from build123d import *

# Parameters (mm, degrees)
SALIENTE_EXTRUIR1_DEPTH = 20
CROQUIS2_R              = 1.75
SALIENTE_EXTRUIR2_DEPTH = 5
MATRIZL1_COUNT          = 2
MATRIZL1_PITCH          = 10
SALIENTE_EXTRUIR3_DEPTH = 3


with BuildPart() as part:
    # Croquis1 → Saliente-Extruir1 (new body)
    with BuildSketch(Plane(origin=(0, 0, 0), x_dir=(1, 0, 0), z_dir=(0, 1, 0))):
        with BuildLine():
            Line((-50.5, 0), (50.5, 0))
            Line((50.5, 0), (50.5, 7))
            Line((50.5, 7), (43.6, 7))
            ThreePointArc((43.6, 7), (31.822793565, 12.849892164), (29.368318159, 25.768846465))
            ThreePointArc((29.368318159, 25.768846465), (25.038732007, 51.41585196), (2.5, 64.397368307))
            Line((2.5, 64.397368307), (2.5, 60.381811917))
            ThreePointArc((2.5, 60.381811917), (0, 7.5), (-2.5, 60.381811917))
            Line((-2.5, 60.381811917), (-2.5, 64.397368307))
            ThreePointArc((-2.5, 64.397368307), (-25.038732007, 51.41585196), (-29.368318159, 25.768846465))
            ThreePointArc((-29.368318159, 25.768846465), (-31.822793565, 12.849892164), (-43.6, 7))
            Line((-43.6, 7), (-50.5, 7))
            Line((-50.5, 7), (-50.5, 0))
        make_face()
        with BuildLine():
            Line((14.186260959, 7), (32.013771293, 7))
            ThreePointArc((32.013771293, 7), (27.872929965, 11.516026639), (25.406103057, 17.124576229))
            ThreePointArc((25.406103057, 17.124576229), (20.433198062, 11.356360342), (14.186260959, 7))
        make_face(mode=Mode.SUBTRACT)
        with BuildLine():
            Line((-32.013771293, 7), (-14.186260959, 7))
            ThreePointArc((-14.186260959, 7), (-20.433198062, 11.356360342), (-25.406103057, 17.124576229))
            ThreePointArc((-25.406103057, 17.124576229), (-27.872929965, 11.516026639), (-32.013771293, 7))
        make_face(mode=Mode.SUBTRACT)
    extrude(amount=SALIENTE_EXTRUIR1_DEPTH)

    # Croquis2 → Saliente-Extruir2 (add)
    with BuildSketch(Plane.ZY.offset(-2.5)):
        with BuildLine():
            Line((-60.381811917, 20), (-60.381811917, 0))
            Line((-60.381811917, 0), (-71.739628608, 0))
            ThreePointArc((-71.739628608, 0), (-76.060720262, 15.678908346), (-60.381811917, 20))
        make_face()
        with Locations((-72.810720262, 10)):
            Circle(CROQUIS2_R, mode=Mode.SUBTRACT)
    saliente_extruir2 = extrude(amount=-SALIENTE_EXTRUIR2_DEPTH)

    # MatrizL1: Saliente-Extruir2 ×2
    with Locations(*[(-i * MATRIZL1_PITCH, 0, 0) for i in range(1, MATRIZL1_COUNT)]):
        add(saliente_extruir2)

    # Croquis3 → Saliente-Extruir3 (add)
    with BuildSketch(Plane(origin=(0, 0, 0), x_dir=(1, 0, 0), z_dir=(0, 1, 0))):
        with BuildLine():
            Line((-7.5, 70.792294373), (-7.5, 63.563490998))
            ThreePointArc((-7.5, 63.563490998), (-20.283716212, 56.7776394), (-28.5, 44.862780491))
            add(Edge.make_bspline(
                [(-7.5, 70.792294373), (-28.5, 65.390312314), (-28.5, 44.862780491)],
                knots=[4.978682998, 4.978682998, 4.978682998, 6.283185307, 6.283185307, 6.283185307], degree=2, weights=[1, 0.794719414, 1]))
        make_face()
        with BuildLine():
            Line((7.5, 70.792294373), (7.5, 63.563490998))
            ThreePointArc((7.5, 63.563490998), (20.283716212, 56.7776394), (28.5, 44.862780491))
            add(Edge.make_bspline(
                [(28.5, 44.862780491), (28.5, 65.390312314), (7.5, 70.792294373)],
                knots=[3.141592654, 3.141592654, 3.141592654, 4.446094963, 4.446094963, 4.446094963], degree=2, weights=[1, 0.794719414, 1]))
        make_face()
    extrude(amount=SALIENTE_EXTRUIR3_DEPTH)


solid = part.part
Work out the finished part from the listing and answer in its coordinate system (mm). A direction names the side the tool comes from. Round coordinates to 2 decimals unless told otherwise and drop trailing zeros. Write each loop counter-clockwise with the first axis right and the second up, starting at its lowest first coordinate (ties: lowest second). Pieces come first, ordered by that corner, then holes.
1) A cutting plane is placed at B-B (y = 10). Give the number of separate pieces and of enclosed holes in the cut face, plus the area to 3 significant figures.
2) The mould has two halves that part along X. Classify faces 6 (the cylindrical face through (-5.04, 10.08, -74.56)), 7 (the flat face through (50.5, 10, -3)), 8 (the cylindrical face through (20.512, 9.86, -11.428)): pulls with the +X half, pulls with the -X half, needs draft (parallel to the pull), parting line crosses it, or undercut.
3) A cutting plane is placed at D-D (y = 15.5). Give the vertices of the cut face in (x, z).
4) Given pin 1 Ø7.5 at (x, y) = (48.5, 11.5) entering from -Z; pin 2 Ø4 at (y, z) = (10, -72.81) entering from +X; pin 3 Ø10.5 at (x, z) = (20.5, -58.5) entering from +Y; pin 4 Ø2 at (y, z) = (10, -72.81) entering from +X, each flat-ended and moving along its own axis, determine where each tip first touches the part or whether it passes through.
5) A cutting plane is placed at A-A (z = -34). Give the vertices of the cut face in (x, y).
6) A tool of negligible diameter and unlimited length cuts with its end or side. For faces 1 (the flat face through (47, 10, -7)), 2 (the flat face through (-2.5, 11, -69)), 3 (the flat face through (7.5, 11, -71)), 4 (the cylindrical face through (1.13, 9.86, -7.524)), 5 (the flat face through (-7.5, 11, -71)), from which of +Z, -Z, +X, -X, +Y, -Y can it reach the whole face along a straight path? Write none if from no direction.
7) A cutting plane is placed at C-C (z = -14.5). Give the vertices of the cut face in (x, y), plus the area to 3 significant figures.
8) Straight lines are drawn through the part: line 1 (X direction, y = 12, z = -34); line 2 (X direction, y = 13.25, z = -9.5); line 3 (Y direction, x = 18.5, z = -6). For each, find the intervals that lie inside material, in ascending order.
Completed:
1. separate pieces: 3
1. enclosed holes: 2
1. area: 1,570 mm2
2. face 6: needs draft
2. face 7: pulls with the +X half
2. face 8: undercut
3. outline: (-50.5, -7) - (-43.6, -7) arc R14.78 cw to (-29.37, -25.77) arc R30.5 ccw to (-7.5, -63.56) - (-7.5, -76.16) - (-2.5, -76.16) - (-2.5, -60.38) arc R26.5 cw (long way) to (2.5, -60.38) - (2.5, -76.16) - (7.5, -76.16) - (7.5, -63.56) arc R30.5 ccw to (29.37, -25.77) arc R14.78 cw to (43.6, -7) - (50.5, -7) - (50.5, 0) - (-50.5, 0) - close; hole (-32.01, -7) arc R18.78 cw to (-25.41, -17.12) arc R30.5 cw to (-14.19, -7) - close; hole (14.19, -7) arc R30.5 cw to (25.41, -17.12) arc R18.78 cw to (32.01, -7) - close
4. pin 1: stops at z = -7
4. pin 2: stops at x = 7.5
4. pin 3: stops at y = 20
4. pin 4: passes through
5. outline: (-30.5, 0) - (-26.5, 0) - (-26.5, 20) - (-30.5, 20) - close; (26.5, 0) - (30.5, 0) - (30.5, 20) - (26.5, 20) - close
6. face 1: -Z, +X, +Y, -Y
6. face 2: -Z, +Y, -Y
6. face 3: -Z, +X, +Y
6. face 4: +Y, -Y
6. face 5: -Z, -X, +Y
7. outline: (-30.74, 0) - (-26.29, 0) - (-26.29, 20) - (-30.74, 20) - close; (-23.45, 0) - (-17.94, 0) - (-17.94, 20) - (-23.45, 20) - close; (17.94, 0) - (23.45, 0) - (23.45, 20) - (17.94, 20) - close; (26.29, 0) - (30.74, 0) - (30.74, 20) - (26.29, 20) - close
7. area: 398 mm2
8. line 1: x = -30.5 to -26.5, 26.5 to 30.5
8. line 2: x = -35.38 to -29.39, -18.17 to -10.1, 10.1 to 18.17, 29.39 to 35.38
8. line 3: y = 0 to 20
